For this review, take the finished solid that the model builds, in its own axes (mm). Face numbers are marked on the shaded views. A direction names the side the tool comes from. Give positions to 0.01 mm unless a question says otherwise; leave off trailing zeros. Order: outer loops, then holes, each group sorted by start corner. A loop starts at its lowest first (then second) coordinate and runs counter-clockwise, first axis right, second up. Notation, with made-up numbers: M -31,-40 L -17,-40 A25 ccw -17,-15 Z; hole C -13.5,27 d4. An arc over 180 degrees is marked long. Use CSV: the item, a comma, the result in double quotes. Start each with the question number.
(1) Consider section A-A (z = -8). Write out the cut boundary in (x, y), and give its area (3 significant figures).
(2) Clearance check with flat-ended pins moving along their axes: P1, Ø6.5, axis at x = 25.5, z = -14, coming from the +Y side; P2, Ø10, axis at x = 23, y = 37, coming from the -Z side; P3, Ø8, axis at y = 24.5, z = -4, coming from the -X side. State where each tip first meets the part, or that it passes through.
(3) Consider section B-B (x = 27.5). Write out the cut boundary in (y, z).
(4) Consider section D-D (x = 7.5). Write out the cut boundary in (y, z), and give its area (3 significant figures).
(5) Tool access review of the marked faces 1 and 2: name each direction out of +Z, -Z, +X, -X, +Y, -Y from which nothing blocks a thin tool from reaching the whole face with its end or side.
(6) Consider section C-C (y = 36.5). Write out the cut boundary in (x, z).
(7) Wall thickness on L1, parallel to X at y = 1.9, z = -8; L2, parallel to Y at x = 29, z = -21.5; L3, parallel to Z at x = 12, y = 18.5: over which ranges is each line inside the solid? List them lowest first. Write a range as from..to.
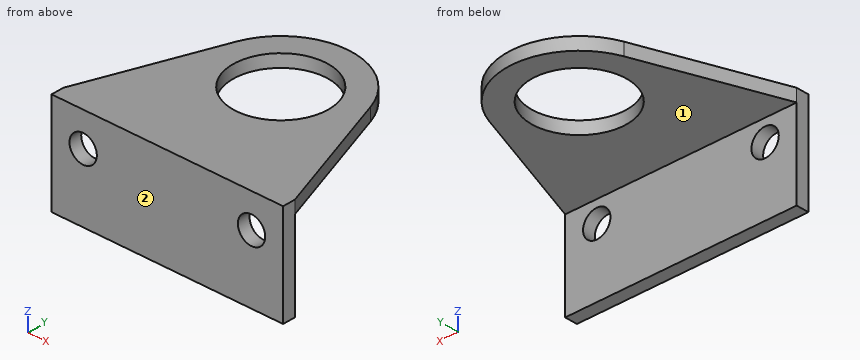
```python
from build123d import *

# Parameters (mm, degrees)
SKETCH_1_W      = 55
SKETCH_1_H      = 24
SKETCH_1_R      = 3.25
EXTRUDE_1_DEPTH = 3
SKETCH_3_R      = 11.25
EXTRUDE_2_DEPTH = 3


with BuildPart() as part:
    # 草图1 → 凸台-拉伸1 (new body)
    with BuildSketch(Plane(origin=(0, 0, 0), x_dir=(1, 0, 0), z_dir=(0, 1, 0))):
        with Locations((27.5, 12)):
            Rectangle(SKETCH_1_W, SKETCH_1_H)
        with Locations(Location((47.5, 8, 0), (0, 0, 270))):
            Circle(SKETCH_1_R, mode=Mode.SUBTRACT)
        with Locations(Location((7.5, 8, 0), (0, 0, 270))):
            Circle(SKETCH_1_R, mode=Mode.SUBTRACT)
    extrude(amount=EXTRUDE_1_DEPTH)

    # 草图3 → 凸台-拉伸2 (add)
    with BuildSketch(Plane.XY):
        with BuildLine():
            Line((0, 3), (11.516480911, 34.790260575))
            ThreePointArc((11.516480911, 34.790260575), (27.5, 46), (43.483519089, 34.790260575))
            Line((43.483519089, 34.790260575), (55, 3))
            Line((55, 3), (0, 3))
        make_face()
        with Locations((27.5, 29)):
            Circle(SKETCH_3_R, mode=Mode.SUBTRACT)
    extrude(amount=-EXTRUDE_2_DEPTH)


solid = part.part
```
Check result:
1,outline,"M 0,0 L 4.25,0 L 4.25,3 L 0,3 Z; M 10.75,0 L 44.25,0 L 44.25,3 L 10.75,3 Z; M 50.75,0 L 55,0 L 55,3 L 50.75,3 Z"
1,area,"126 mm^2"
2,P1,"stops at y = 3"
2,P2,"stops at z = -3"
2,P3,"stops at x = 6.39"
3,outline,"M 0,-24 L 3,-24 L 3,-3 L 17.75,-3 L 17.75,0 L 0,0 Z; M 40.25,-3 L 46,-3 L 46,0 L 40.25,0 Z"
4,outline,"M 0,-24 L 3,-24 L 3,-11.25 L 0,-11.25 Z; M 0,-4.75 L 3,-4.75 L 3,-3 L 23.7,-3 L 23.7,0 L 0,0 Z"
4,area,"115 mm^2"
5,face 1,"-Z, +X, -X, +Y"
5,face 2,"+Z, -Z, +X, -X, -Y"
6,outline,"M 12.24,-3 L 19.11,-3 L 19.11,0 L 12.24,0 Z; M 35.89,-3 L 42.76,-3 L 42.76,0 L 35.89,0 Z"
7,L1,"x = 0..4.25, 10.75..44.25, 50.75..55"
7,L2,"y = 0..3"
7,L3,"z = -3..0"
